Autodesk Inventor part; units mm, degrees
ref_plane "Work Plane1" through (-15, 0, -10) normal (0, 0, 1) x (0, 1, 0)
ref_plane "YZ Plane" through (0, 0, 0) normal (1, 0, 0) x (0, 1, 0)
ref_plane "XZ Plane" through (0, 0, 0) normal (0, 1, 0) x (-1, 0, 0)
sketch "Sketch1" plane through (0, 0, 0) normal (0, 1, 0) x (-1, 0, 0)
  circle A0 centre (0, 0) radius 5
  line L0 (-23.6, 0) -> (36.6, 0) construction
  line L1 (0, -52.2) -> (0, 61.2) construction
  circle A1 centre (0, 20) radius 5.125
  circle A2 centre (0, -20) radius 5.125
  circle A3 centre (-10, 0) radius 2
  circle A4 centre (11, 24) radius 2
  line L2 (0, 45) -> (15, 30)
  line L3 (15, 30) -> (15, -10)
  line L4 (15, -10) -> (28, -23)
  line L5 (28, -23) -> (28, -36)
  line L6 (28, -36) -> (-15, -36)
  line L7 (-15, -36) -> (-15, 45)
  line L8 (-15, 45) -> (0, 45)
  line L9 (0.375, 14.8887) -> (0.375, 8.8887)
  line L10 (0.375, 8.8887) -> (-0.375, 8.8887)
  line L11 (-0.375, 8.8887) -> (-0.375, 14.8887)
  line L12 (0.375, -14.8887) -> (0.375, -8.8887)
  line L13 (0.375, -8.8887) -> (-0.375, -8.8887)
  line L14 (-0.375, -8.8887) -> (-0.375, -14.8887)
  dimension "d0" = 10
  dimension "d1" = 10.25
  dimension "d3" = 40
  dimension "d4" = 4
  dimension "d5" = 11
  dimension "d6" = 4
  dimension "d9" = 10
  dimension "d10" = 4
  dimension "d13" = 45
  dimension "d14" = 15
  dimension "d16" = 16
  dimension "d17" = 13
  dimension "d18" = 45
  dimension "d19" = 25
  dimension "d24" = 0.75
  dimension "d25" = 6
  dimension "d106" = 13
extrude "Extrusion1" add sketch "Sketch1" along normal blind 40
sketch "Sketch2" plane through (0, 0, 0) normal (0, -1, 0) x (1, 0, 0)
  circle A0 centre (0, 0) radius 5
extrude "Extrusion2" add sketch "Sketch2" against normal blind 20
sketch "Sketch3" plane through (0, 0, 0) normal (0, -1, 0) x (1, 0, 0)
  arc A0 (-0.375, -14.8887) -> (0.375, -14.8887) centre (0, -20) ccw
  circle A1 centre (0, -20) radius 2.5
  line L0 (-36.6, 0) -> (23.6, 0) construction
  line L1 (0.375, -14.8887) -> (0.375, -8.8887)
  line L2 (-0.375, -8.8887) -> (-0.375, -14.8887)
  line L3 (0.375, -8.8887) -> (-0.375, -8.8887)
  line L4 (-0.375, -14.8887) -> (-0.375, -17.5283)
  line L5 (0.375, -14.8887) -> (0.375, -17.5283)
  line L6 (-0.375, -22.4717) -> (-0.375, -24.9717)
  line L7 (-0.375, -24.9717) -> (0.375, -24.9717)
  line L8 (0.375, -24.9717) -> (0.375, -22.4717)
  arc A2 (0.375, 14.8887) -> (-0.375, 14.8887) centre (0, 20) ccw
  line L9 (-0.375, 14.8887) -> (-0.375, 8.8887)
  line L10 (0.375, 8.8887) -> (0.375, 14.8887)
  line L11 (-0.375, 8.8887) -> (0.375, 8.8887)
  circle A3 centre (0, 20) radius 2.5
  line L12 (-0.375, 14.8887) -> (-0.375, 17.5283)
  line L13 (0.375, 14.8887) -> (0.375, 17.5283)
  line L14 (-0.375, 22.4717) -> (-0.375, 24.9717)
  line L15 (-0.375, 24.9717) -> (0.375, 24.9717)
  line L16 (0.375, 24.9717) -> (0.375, 22.4717)
  line L17 (-0.375, -8.8887) -> (-0.375, -14.8887)
  arc A4 (0.375, -14.8887) -> (-0.375, -14.8887) centre (0, -20) ccw
  arc A5 (-0.375, 14.8887) -> (0.375, 14.8887) centre (0, 20) ccw
  point P0 (0, 0)
  dimension "d26" = 5
  dimension "d27" = 2.5
  dimension "d30" = 5.125
  dimension "d31" = 5.125
extrude "Extrusion3" add sketch "Sketch3" against normal blind 3.5 contours L4 A1 L6 L7 L8 L5 A0 | L2 L3 L1 A4 | L13 A3 L16 L15 L14 L12 A2 | L10 L11 L9 A5
sketch "Sketch4" plane through (15, 0, 45) normal (1, 0, 0) x (0, 0, -1)
  line L0 (81, 0) -> (81, 40) construction
  line L1 (81, 33.145) -> (85.85, 33.145)
  line L2 (86.85, 32.145) -> (86.85, 27.855)
  line L3 (85.85, 26.855) -> (81, 26.855)
  line L4 (81, 26.855) -> (81, 33.145)
  line L5 (81, 20) -> (108.6331, 20) construction
  line L6 (0, 40) -> (81, 40) construction
  line L7 (85.85, 33.145) -> (86.85, 32.145)
  line L8 (85.85, 26.855) -> (86.85, 27.855)
  line L9 (81, 6.855) -> (85.85, 6.855)
  line L10 (86.85, 7.855) -> (86.85, 12.145)
  line L11 (85.85, 13.145) -> (81, 13.145)
  line L12 (81, 13.145) -> (81, 6.855)
  line L13 (85.85, 6.855) -> (86.85, 7.855)
  line L14 (85.85, 13.145) -> (86.85, 12.145)
  point P0 (45, 0)
  point P1 (86.85, 26.855)
  point P2 (86.85, 33.145)
  point P3 (86.85, 13.145)
  point P4 (86.85, 6.855)
  dimension "d32" = 6.855
  dimension "d33" = 5.85
  dimension "d34" = 6.29
  dimension "d35" = 1
  dimension "d36" = 1
  dimension "d37" = 1
  dimension "d38" = 1
extrude "Extrusion4" add sketch "Sketch4" against normal up to surface (43 mm away)
sketch "Sketch5" plane through (15, 27.855, -41.85) normal (0, 0, -1) x (-1, 0, 0)
  line L0 (30, -27.855) -> (30, 12.145) construction
  line L1 (0, 5.29) -> (43, 5.29)
  line L2 (36, 5.29) -> (36, -1) construction
  line L3 (43, -1) -> (0, -1)
  circle A0 centre (36, 2.145) radius 2.25
  line L4 (0, -27.855) -> (0, 12.145)
  line L5 (0, -7.855) -> (43, -7.855) construction
  line L6 (43, -27.855) -> (43, 12.145)
  circle A1 centre (36, -17.855) radius 2.25
  point P0 (15, -27.855)
  dimension "d41" = 4.5
  dimension "d42" = 6
extrude "Extrusion5" cut sketch "Sketch5" against normal through all contours A0 | A1
ref_plane "Work Plane1" through (-15, 0, -10) normal (0, 0, 1) x (0, 1, 0)
sketch "Sketch6" plane through (-15, 0, -10) normal (0, 0, 1) x (0, 1, 0)
  circle A0 centre (30, 6) radius 2.25
  circle A1 centre (30, 6) radius 3.75
  circle A2 centre (10, 6) radius 2.25
  circle A3 centre (10, 6) radius 3.75
  point P0 (0, -15)
  dimension "d46" = 7.5
  dimension "d47" = 7.5
extrude "Extrusion6" cut sketch "Sketch6" against normal blind 21 contours A0 | A1 | A2 | A3
sketch "Sketch7" plane through (15, 27.855, -41.85) normal (0, 0, -1) x (-1, 0, 0)
  line L0 (0, -27.855) -> (0, 12.145)
  line L1 (0, -7.855) -> (43, -7.855) construction
  line L2 (43, -27.855) -> (43, 12.145)
  line L3 (0, -15.71) -> (0, -20)
  line L4 (0, -12.855) -> (-10, -12.855)
  line L5 (-10, -12.855) -> (-10, -27.855)
  line L6 (-10, -27.855) -> (0, -27.855)
  line L7 (0, -27.855) -> (0, -12.855)
  line L8 (15, -27.855) -> (0, -27.855)
  point P0 (0, 0)
  point P1 (0, 4.29)
  point P2 (0, -17.855)
  point P3 (0, -12.855)
  point P4 (-10, -20.355)
  dimension "d63" = 10
  dimension "d64" = 5
extrude "Extrusion7" add sketch "Sketch7" against normal up to surface (86.85 mm away)
sketch "Sketch9" plane through (-28, 27.855, -41.85) normal (0, 0, -1) x (-1, 0, 0)
  arc A0 (-6.3207, 0) -> (-6.3207, 4.29) centre (-7, 2.145) ccw
  line L0 (-43, -6.9275) -> (0, -7.855) construction
  line L1 (0, -14.71) -> (0, -1)
  circle A1 centre (-48, -17.855) radius 2.25
  line L2 (-43, -12.855) -> (-53, -12.855)
  arc A2 (-7.6793, -15.71) -> (-7.6793, -20) centre (-7, -17.855) ccw
  line L3 (-7, -17.855) -> (-48, -17.855) construction
  line L4 (-48, -12.855) -> (-48, -17.855) construction
  point P0 (-28, -27.855)
extrude "Extrusion9" cut sketch "Sketch9" against normal through all
sketch "Sketch10" plane through (0, 0, 45) normal (0, 0, 1) x (1, 0, 0)
  circle A0 centre (20, 10) radius 2.25
  circle A1 centre (20, 10) radius 3.5
  point P0 (0, 0)
  dimension "d59" = 7
extrude "Extrusion10" cut sketch "Sketch10" against normal blind 70 contours A0 | A1
sketch "Sketch11" plane through (25, 0, -41.85) normal (1, 0, 0) x (0, 0, -1)
  line L0 (-1, 13.145) -> (-5.85, 13.145)
  line L1 (-5.85, 13.145) -> (-5.85, 15)
  line L2 (0, 15) -> (-5.85, 15)
  line L3 (0, 12.145) -> (0, 15)
  line L4 (0, 12.145) -> (-1, 13.145)
  line L5 (-5.85, 13.145) -> (-5.85, 6.855)
  line L6 (0, 0) -> (0, 7.855)
  line L7 (-1, 6.855) -> (0, 7.855)
  line L8 (-5.85, 6.855) -> (-1, 6.855)
  line L9 (-5.85, 0) -> (-5.85, 6.855)
  line L10 (-5.85, 6.855) -> (-5.85, 0)
  line L11 (0, 0) -> (-86.85, 0)
  line L12 (-5.85, 0) -> (0, 0)
  point P0 (-41.85, 0)
extrude "Extrusion11" cut sketch "Sketch11" against normal through all
sketch "Sketch12" plane through (15, 27.855, -41.85) normal (1, 0, 0) x (0, 0, -1)
  line L0 (-43.85, 12.145) -> (-39.85, 12.145)
  line L1 (-44.85, -27.855) -> (-38.85, -27.855)
  line L2 (-38.85, -27.855) -> (-38.85, 2.145)
  line L3 (-38.85, 2.145) -> (-44.85, 2.145)
  line L4 (-44.85, 2.145) -> (-44.85, -27.855)
  line L5 (-41.85, 12.145) -> (-41.85, 2.145)
  line L6 (-31.85, -27.855) -> (-71.85, -27.855)
  point P0 (-41.85, -27.855)
  dimension "d72" = 10
  dimension "d74" = 6
extrude "Extrusion12" cut sketch "Sketch12" against normal blind 8
sketch "Sketch13" plane through (-15, 10, -10) normal (-1, 0, 0) x (0, 0, 1)
  line L0 (32, 30) -> (36, 30)
  line L1 (34, 30) -> (34, 20)
  line L2 (31, -10) -> (37, -10)
  line L3 (37, -10) -> (37, 20)
  line L4 (37, 20) -> (31, 20)
  line L5 (31, 20) -> (31, -10)
  line L6 (0, -10) -> (40, -10)
  dimension "d79" = 6
  dimension "d110" = 10
extrude "Extrusion13" cut sketch "Sketch13" against normal blind 8
chamfer "Chamfer2" distance 13 distance2 5 1 edges at (-28, 40, -29.5) measured on face at (-4.5425, 40, -32.3621)
chamfer "Chamfer3" distance 6 angle 45 1 edges at (-28, 0, -29.5)
sketch "Sketch18" plane through (15, 15, -36) normal (0, 1, 0) x (1, 0, 0)
  line L0 (-37, -19) -> (-43, -13) construction
  line L1 (10, 0) -> (10, -81)
  line L2 (0, -81) -> (0, 0)
  line L3 (10, 0) -> (0, 0)
  line L4 (0, 0) -> (0, -5)
  line L5 (0, -5) -> (10, -5)
  line L6 (10, -5) -> (10, 0)
  line L7 (10, 0) -> (10, -81)
  line L8 (10, -81) -> (0, -81)
  line L9 (8.5, -81) -> (1.5, -81)
  point P0 (-15, -36)
  point P1 (10, -5)
  dimension "d109" = 5
extrude "Extrusion18" cut sketch "Sketch18" against normal through all contours L1 L8 L2 L5
sketch "Sketch20" plane through (0, 40, 0) normal (0, 1, 0) x (1, 0, 0)
  line L0 (17.75, 41.85) -> (22.25, 41.85)
  line L1 (-20.3207, 41.85) -> (-18.75, 41.85)
  line L2 (25, 36) -> (15, 36)
  line L3 (15, 36) -> (15, 41.85)
  line L4 (15, 41.85) -> (25, 41.85)
  line L5 (25, 41.85) -> (25, 36)
  line L6 (25, 40.85) -> (25, 36)
  line L7 (25, 36) -> (15, 36)
  line L8 (25, 41.85) -> (-28, 41.85) construction
  line L9 (15, 40.85) -> (15, 36)
  line L10 (-28, 41.85) -> (-15, 41.85)
  line L11 (-15, 41.85) -> (-15, 36)
  line L12 (-15, 36) -> (-28, 36)
  line L13 (-28, 36) -> (-28, 41.85)
  line L14 (-15, 36) -> (-28, 36)
  line L15 (-28, 40.85) -> (-28, 36)
  line L16 (15, 41.85) -> (-28, 41.85) construction
  line L17 (-15, 10) -> (-15, 36)
  point P0 (0, 0)
extrude "Extrusion19" cut sketch "Sketch20" against normal through all
equation "\"d30\" = d31"
equation "\"d47\" = d46"
equation "\"d79\" = d74"
properties part number "_3DPrint"
The model under review builds one solid part; all positions refer to its coordinate system, in mm. A direction names the side the tool comes from. Round coordinates to 2 decimals unless told otherwise and drop trailing zeros. Order: outer loops, then holes, each group sorted by start corner. A loop starts at its lowest first (then second) coordinate and runs counter-clockwise, first axis right, second up. Notation, with made-up numbers: M -18.75,32.25 L 1.25,32.25 A4 ccw 1.25,39.25 Z; hole C -10,-17.75 d4. An arc over 180 degrees is marked long. Use a Markdown table: item, result.
1) Wall thickness on line 1 along Z through (x, y) = (0, 17) (3 decimals); line 2 along Z through (x, y) = (-10, 17); line 3 along Z through (x, y) = (9, 16.5): over which ranges is each line inside the solid? List them lowest first. Write a range as [from, to].
Report:
| item | result |
|---|---|
| line 1 | [-36, -25.125], [-8.889, 8.889], [25.125, 45] |
| line 2 | [-36, 21], [27, 35] |
| line 3 | [-36, -3], [3, 45] |
2) Insertion check: pin 1 (7 mm diameter, centred on x = -21, y = 10, fed in from -Z); pin 2 (1.5 mm diameter, centred on x = -2, z = -39.5, fed in from -Y) (3 decimals); pin 3 (3 mm diameter, centred on y = 7.5, z = 19, fed in from -X). Each pin has a flat end and moves straight along its axis. Give the tip position at first contact, or say it passes through.
Report:
| item | result |
|---|---|
| pin 1 | z = -36 |
| pin 2 | y = 6.855 |
| pin 3 | x = -15 |
3) Tool access review of faces 4 (the face through (11, 15, -3)), 5 (the face through (0, 26.855, -38)), 6 (the face through (-15, 20, 10)), 7 (the face through (-19, 12, -31)): name each direction out of +Z, -Z, +X, -X, +Y, -Y from which nothing blocks a thin tool from reaching the whole face with its end or side.
Report:
| item | result |
|---|---|
| face 4 | +X, -Y |
| face 5 | -Z, +X, -X |
| face 6 | +Z, -X, +Y, -Y |
| face 7 | +Z |
4) Draft analysis for pull direction X (two halves, no side actions). For faces 1 (the face through (7, 15, 0)), 2 (the face through (-28, 20, -29)), 3 (the face through (0.375, 2, -16)), state which applies: released by +X, released by -X, zero draft, split by the parting line, or undercut.
Report:
| item | result |
|---|---|
| face 1 | released by +X |
| face 2 | released by -X |
| face 3 | undercut |
5) Consider section C-C (z = -18.5). Write out the cut boundary in (x, y).
Report:
| item | result |
|---|---|
| outline | M -23.5,1.5 L -22,0 L -2,0 L -2,3.5 L -4.9,3.5 L -4.9,40 L -15,40 L -23.5,36.73 L -23.5,32.8 A3.75 cw long -23.5,27.2 L -23.5,12.8 A3.75 cw long -23.5,7.2 Z; M 2,0 L 15,0 L 15,40 L 4.9,40 L 4.9,3.5 L 2,3.5 Z |
6) Consider section D-D (y = 24). Write out the cut boundary in (x, z) (3 decimals), then the cut area to 3 significant figures.
Report:
| item | result |
|---|---|
| outline | M -28,-36 L 15,-36 L 15,-3 L 7,-3 L 7,3 L 15,3 L 15,45 L 0,45 L -15,30 L -15,27 L -7,27 L -7,21 L -15,21 L -15,-10 L -28,-23 Z; hole C 0,0 d10; hole M -0.375,-14.889 A5.125 ccw long 0.375,-14.889 L 0.375,-8.889 L -0.375,-8.889 Z; hole M -0.375,8.889 L 0.375,8.889 L 0.375,14.889 A5.125 ccw long -0.375,14.889 Z |
| area | 2,220 mm^2 |
7) Consider section A-A (x = 10). Write out the cut boundary in (y, z) (3 decimals), then the cut area to 3 significant figures.
Report:
| item | result |
|---|---|
| outline | M 0,-36 L 6.855,-36 L 6.855,-40.85 L 7.855,-41.85 L 12.145,-41.85 L 13.145,-40.85 L 13.145,-36 L 26.855,-36 L 26.855,-40.85 L 27.855,-41.85 L 32.145,-41.85 L 33.145,-40.85 L 33.145,-36 L 40,-36 L 40,-2 L 30,-2 L 30,-3 L 0,-3 Z; M 0,3 L 30,3 L 30,2 L 40,2 L 40,45 L 0,45 Z |
| area | 3,090 mm^2 |
8) Consider section B-B (y = 18.5). Write out the cut boundary in (x, z) (3 decimals).
Report:
| item | result |
|---|---|
| outline | M -28,-36 L 15,-36 L 15,-3 L 7,-3 L 7,3 L 15,3 L 15,45 L 0,45 L -15,30 L -15,27 L -7,27 L -7,21 L -15,21 L -15,-10 L -28,-23 Z; hole M -0.375,-14.889 A5.125 ccw long 0.375,-14.889 L 0.375,-8.889 L -0.375,-8.889 Z; hole M -0.375,8.889 L 0.375,8.889 L 0.375,14.889 A5.125 ccw long -0.375,14.889 Z |
